```python
from build123d import *

# Parameters (mm, degrees)
SKETCH1_W           = 32.75
SKETCH1_H           = 26.9
BOSS_EXTRUDE1_DEPTH = 3.25
FILLET1_R           = 3
SKETCH2_R           = 5
SKETCH2_R_2         = 1.6
CUT_EXTRUDE1_DEPTH  = 3.25
SKETCH4_W           = 3.25
SKETCH4_H           = 26.9
BOSS_EXTRUDE2_DEPTH = 30.75
FILLET2_R           = 3
SKETCH5_R           = 4
SKETCH5_R_2         = 1.6
CUT_EXTRUDE2_DEPTH  = 30.75
FILLET4_R           = 13


with BuildPart() as part:
    # Sketch1 → Boss-Extrude1 (new body)
    with BuildSketch(Plane.XY):
        with Locations((16.375, 13.45)):
            Rectangle(SKETCH1_W, SKETCH1_H)
    extrude(amount=BOSS_EXTRUDE1_DEPTH)

    # Fillet1
    fillet1_edges = [part.edges().sort_by_distance(p)[0] for p in [
        (32.75, 26.9, 1.625),
        (32.75, 0, 1.625),
    ]]
    fillet(fillet1_edges, radius=FILLET1_R)

    # Sketch2 → Cut-Extrude1 (cut)
    with BuildSketch(Plane.XY.offset(3.25)):
        with BuildLine():
            ThreePointArc((12.35, 21.45), (9.61862915, 22.58137085), (10.75, 19.85))
            Line((10.75, 19.85), (10.75, 21.45))
            Line((10.75, 21.45), (12.35, 21.45))
        make_face()
        with BuildLine():
            Line((10.75, 21.45), (10.75, 19.85))
            ThreePointArc((10.75, 19.85), (11.88137085, 20.31862915), (12.35, 21.45))
            Line((12.35, 21.45), (10.75, 21.45))
        make_face()
        with Locations((17.75, 13.45)):
            Circle(SKETCH2_R)
        with Locations((24.75, 21.45)):
            Circle(SKETCH2_R_2)
        with Locations((24.75, 5.45)):
            Circle(SKETCH2_R_2)
        with Locations((10.75, 5.45)):
            Circle(SKETCH2_R_2)
    extrude(amount=-CUT_EXTRUDE1_DEPTH, mode=Mode.SUBTRACT)

    # Sketch4 → Boss-Extrude2 (add)
    with BuildSketch(Plane(origin=(0, 0, 0), x_dir=(-1, 0, 0), z_dir=(0, 0, -1))):
        with Locations((-1.625, 13.45)):
            Rectangle(SKETCH4_W, SKETCH4_H)
    extrude(amount=BOSS_EXTRUDE2_DEPTH)

    # Fillet2
    fillet2_edges = [part.edges().sort_by_distance(p)[0] for p in [
        (0, 13.45, 3.25),
    ]]
    fillet(fillet2_edges, radius=FILLET2_R)

    # Sketch5 → Cut-Extrude2 (cut)
    with BuildSketch(Plane(origin=(3.25, 0, 0), x_dir=(0, 0, -1), z_dir=(1, 0, 0))):
        with Locations((17.75, 13.45)):
            Circle(SKETCH5_R)
        with Locations((17.75, 21.95)):
            Circle(SKETCH5_R_2)
        with Locations((17.75, 4.95)):
            Circle(SKETCH5_R_2)
    extrude(amount=-CUT_EXTRUDE2_DEPTH, mode=Mode.SUBTRACT)

    # Fillet4
    fillet4_edges = [part.edges().sort_by_distance(p)[0] for p in [
        (1.625, 26.9, -30.75),
        (1.625, 0, -30.75),
    ]]
    fillet(fillet4_edges, radius=FILLET4_R)


solid = part.part
```
Read the model definition and answer for the solid it produces. Units are mm, in the model's axes. A direction names the side the tool comes from. Round coordinates to 2 decimals unless told otherwise and drop trailing zeros. Write each loop counter-clockwise with the first axis right and the second up, starting at its lowest first coordinate (ties: lowest second). Pieces come first, ordered by that corner, then holes. Notation, with made-up numbers: (78, -4) -> (89, -4) arc R14 cw to (89, 4) -> close; hole circle Ø1 at (-30, 86.5). An arc over 180 degrees is marked (long way). Answer in a Markdown table with one row per item. Add a question column.
1) Find section C-C, the plane y = 5.45. Determine the outline of the cut face in (x, z), and give its area (3 significant figures).
2) Find section D-D, the plane y = 11.25. Determine the outline of the cut face in (x, z).
3) Find section B-B, the plane x = 17.75. Determine the outline of the cut face in (y, z), and give its area (3 significant figures).
4) Find section A-A, the plane x = 24.75. Determine the outline of the cut face in (y, z), and give its area (3 significant figures).
5) Which of the six approach directions +Z, -Z, +X, -X, +Y, -Y give full straight-line access (tool end or side, diameter ignored) to faces 5 (the face through (32.75, 13, 2)), 6 (the face through (18, 8, 0))?
6) Determine the mould class of faces 1 (the face through (11, 26.9, 1)), 2 (the face through (1.65, 20.98, -16.48)), 3 (the face through (3.25, 13, -12)), 4 (the face through (24.4, 19.89, 1.65)) for opening direction Y: pulls with the +Y half, pulls with the -Y half, needs draft (parallel to the pull), parting line crosses it, or undercut.
7) Given P1, Ø4, axis at y = 4.95, z = -17.75, coming from the -X side; P2, Ø4, axis at y = 21.95, z = -17.75, coming from the +X side; P3, Ø1, axis at x = 12.5, y = 20.5, coming from the -Z side; P4, Ø6, axis at x = 17.75, y = 13.45, coming from the -Z side, each flat-ended and moving along its own axis, determine where each tip first touches the part or whether it passes through.
8) Consider line 1 (Y direction, x = 10.75, z = 1); line 2 (Y direction, x = 10, z = 2); line 3 (X direction, y = 10.25, z = -23.5). Determine where each line is inside the solid, lowest interval first.
Findings below:
| question | item | result |
|---|---|---|
| 1 | outline | (0, -28.33) -> (3.25, -28.33) -> (3.25, -19.27) -> (0, -19.27) -> close; (0, -16.23) -> (3.25, -16.23) -> (3.25, 0) -> (9.15, 0) -> (9.15, 3.25) -> (3, 3.25) arc R3 ccw to (0, 0.25) -> close; (12.35, 0) -> (23.15, 0) -> (23.15, 3.25) -> (12.35, 3.25) -> close; (26.35, 0) -> (32.75, 0) -> (32.75, 3.25) -> (26.35, 3.25) -> close |
| 1 | area | 166 mm² |
| 2 | outline | (0, -30.63) -> (3.25, -30.63) -> (3.25, -21.09) -> (0, -21.09) -> close; (0, -14.41) -> (3.25, -14.41) -> (3.25, 0) -> (13.26, 0) -> (13.26, 3.25) -> (3, 3.25) arc R3 ccw to (0, 0.25) -> close; (22.24, 0) -> (32.75, 0) -> (32.75, 3.25) -> (22.24, 3.25) -> close |
| 3 | outline | (0, 0) -> (8.45, 0) -> (8.45, 3.25) -> (0, 3.25) -> close; (18.45, 0) -> (26.9, 0) -> (26.9, 3.25) -> (18.45, 3.25) -> close |
| 3 | area | 54.9 mm² |
| 4 | outline | (0, 0) -> (3.85, 0) -> (3.85, 3.25) -> (0, 3.25) -> close; (7.05, 0) -> (19.85, 0) -> (19.85, 3.25) -> (7.05, 3.25) -> close; (23.05, 0) -> (26.9, 0) -> (26.9, 3.25) -> (23.05, 3.25) -> close |
| 4 | area | 66.6 mm² |
| 5 | face 5 | +Z, -Z, +X, +Y, -Y |
| 5 | face 6 | -Z, +X, +Y, -Y |
| 6 | face 1 | pulls with the +Y half |
| 6 | face 2 | undercut |
| 6 | face 3 | needs draft |
| 6 | face 4 | undercut |
| 7 | P1 | x = 0 |
| 7 | P2 | x = 3.25 |
| 7 | P3 | z = 0 |
| 7 | P4 | through |
| 8 | line 1 | 0 to 3.85, 7.05 to 19.85, 23.05 to 26.9 |
| 8 | line 2 | 0 to 4.04, 6.86 to 20.04, 22.86 to 26.9 |
| 8 | line 3 | 0 to 3.25 |
